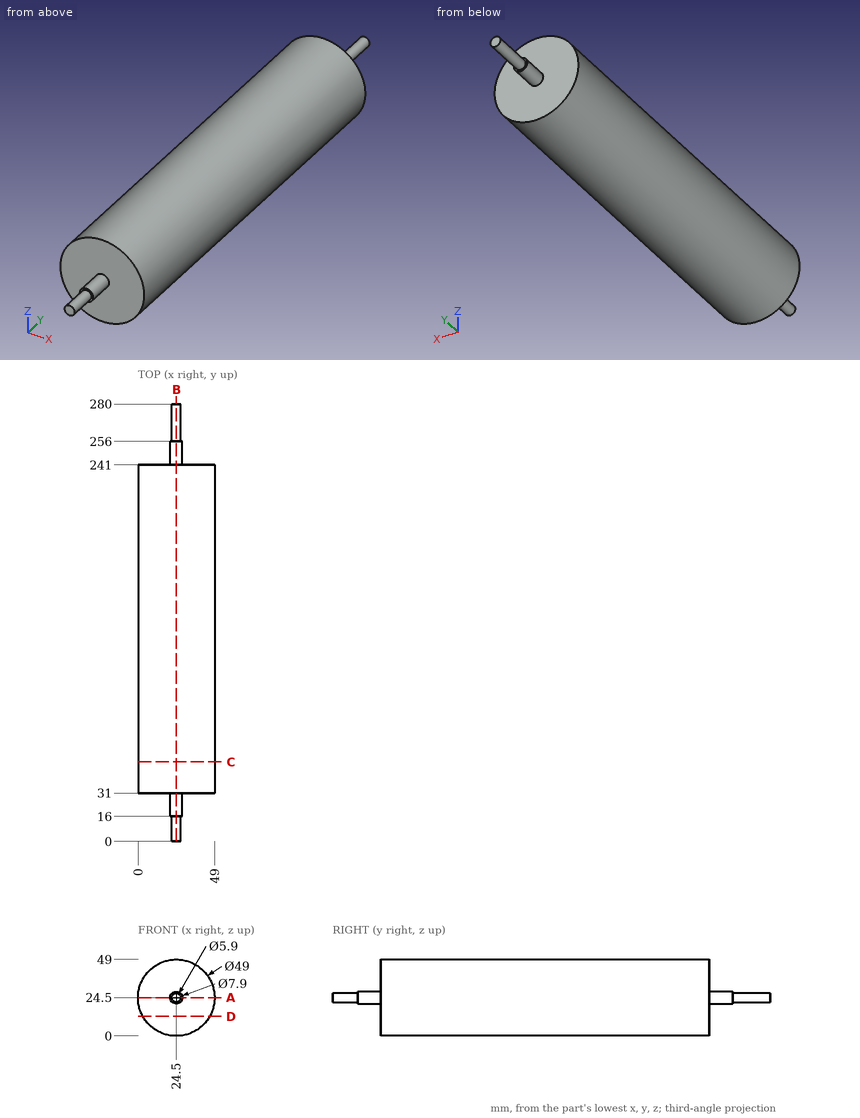
Answer from the drawing. Dimensions are ordinates in mm from the lowest x, y and z of the part. Round coordinates to 2 decimals unless told otherwise and drop trailing zeros. Write each loop counter-clockwise with the first axis right and the second up, starting at its lowest first coordinate (ties: lowest second). Pieces come first, ordered by that corner, then holes. Notation, with made-up numbers: (-29.75, 63) - (-0.75, 63) arc R10 cw to (-0.75, 81) - close; hole circle Ø10 at (25, -12.5). An arc over 180 degrees is marked (long way). One line per item, written item: value.
Q1. Find section D-D (z = 12.5). Determine the outline of the cut face in (x, y), and give its area (3 significant figures).
The answers:
outline: (3.14, 31) - (45.86, 31) - (45.86, 241) - (3.14, 241) - close
area: 8,970 mm2
Q2. Straight lines are drawn through the part: line 1 (Z direction, x = 26, y = 192); line 2 (Y direction, x = 41, z = 33.5); line 3 (X direction, y = 135, z = 23.5). For each, find the intervals that lie inside material, in ascending order. Write a range as from..to.
The answers:
line 1: z = 0.05..48.95
line 2: y = 31..241
line 3: x = 0.02..48.98
Q3. Each of these flat-tipped pins is pushed along its axis until it touches: P1, Ø1.5, axis at x = 23.5, y = 216, coming from the -Z side; P2, Ø1, axis at x = 9.5, y = 221.5, coming from the +Z side; P3, Ø10, axis at x = 37.5, z = 38.5, coming from the +Y side. Where does it stop, or does it pass through?
The answers:
P1: stops at z = 0
P2: stops at z = 44.25
P3: stops at y = 241
Q4. Find section A-A (z = 24.5). Determine the outline of the cut face in (x, y), and give its area (3 significant figures).
The answers:
outline: (0, 31) - (20.55, 31) - (20.55, 16) - (21.55, 16) - (21.55, 0) - (27.45, 0) - (27.45, 16) - (28.45, 16) - (28.45, 31) - (49, 31) - (49, 241) - (28.45, 241) - (28.45, 256) - (27.45, 256) - (27.45, 280) - (21.55, 280) - (21.55, 256) - (20.55, 256) - (20.55, 241) - (0, 241) - close
area: 10,800 mm2
Q5. Find section C-C (y = 51). Determine the outline of the cut face in (x, z).
The answers:
outline: circle Ø49 at (24.5, 24.5)
Q6. Find section B-B (x = 24.5). Determine the outline of the cut face in (y, z).
The answers:
outline: (0, 21.55) - (16, 21.55) - (16, 20.55) - (31, 20.55) - (31, 0) - (241, 0) - (241, 20.55) - (256, 20.55) - (256, 21.55) - (280, 21.55) - (280, 27.45) - (256, 27.45) - (256, 28.45) - (241, 28.45) - (241, 49) - (31, 49) - (31, 28.45) - (16, 28.45) - (16, 27.45) - (0, 27.45) - close
